Verification items for the finished model (mm, model axes). A direction names the side the tool comes from. Coordinates: 2 decimals unless noted, no trailing zeros. Order: outer loops, then holes, each group sorted by start corner. A loop starts at its lowest first (then second) coordinate and runs counter-clockwise, first axis right, second up. Notation, with made-up numbers: (54, -11) - (105, -11) arc R20 cw to (105, 2) - close; hole circle Ø9 at (41, 4.5). An arc over 180 degrees is marked (long way). One line per question, with ' | ' between items. Start each with the question number.
from build123d import *

# Parameters (mm, degrees)
SKETCH1_R           = 3
BOSS_EXTRUDE1_DEPTH = 29
CUT_EXTRUDE1_START  = -3
CUT_EXTRUDE1_DEPTH  = 3
FILLET1_R           = 1


with BuildPart() as part:
    # Sketch1 → Boss-Extrude1 (new body)
    with BuildSketch(Plane.XY):
        with Locations(Location((0, 0, 0), (0, 0, 180))):
            Circle(SKETCH1_R)
    extrude(amount=BOSS_EXTRUDE1_DEPTH)

    # Sketch3 → Cut-Extrude1 (cut)
    with BuildSketch(Plane.XY.offset(29).offset(CUT_EXTRUDE1_START)):
        with BuildLine():
            Line((-3, 0), (-1.5, 2.598076211))
            ThreePointArc((-1.5, 2.598076211), (-2.598076211, 1.5), (-3, 0))
        make_face()
        with BuildLine():
            Line((1.5, 2.598076211), (3, 0))
            ThreePointArc((3, 0), (2.598076211, 1.5), (1.5, 2.598076211))
        make_face()
        with BuildLine():
            Line((-1.5, 2.598076211), (1.5, 2.598076211))
            ThreePointArc((1.5, 2.598076211), (0, 3), (-1.5, 2.598076211))
        make_face()
        with BuildLine():
            ThreePointArc((-3, 0), (-2.598076211, -1.5), (-1.5, -2.598076211))
            Line((-1.5, -2.598076211), (-3, 0))
        make_face()
        with BuildLine():
            ThreePointArc((-1.5, -2.598076211), (0, -3), (1.5, -2.598076211))
            Line((1.5, -2.598076211), (-1.5, -2.598076211))
        make_face()
        with BuildLine():
            ThreePointArc((1.5, -2.598076211), (2.598076211, -1.5), (3, 0))
            Line((3, 0), (1.5, -2.598076211))
        make_face()
    cut_extrude1 = extrude(amount=CUT_EXTRUDE1_DEPTH, mode=Mode.SUBTRACT)

    # Mirror1: Cut-Extrude1 across plane
    add(cut_extrude1.mirror(Plane(origin=(0, 0, 14.5), x_dir=(1, 0, 0), z_dir=(0, 0, -1))), mode=Mode.SUBTRACT)

    # Sketch6 → Tap Drill for M3x0.5 Tap1 (revolve, cut)
    with BuildSketch(Plane(origin=(0, 0, 29), x_dir=(0, -1, 0), z_dir=(1, 0, 0))):
        Polygon((0, 0), (0, 5.751075774), (1.25, 5), (1.25, 0), align=None)
    tap_drill_for_m3x0_5_tap1 = revolve(axis=Axis((0, 0, 35.35), (0, 0, -1)), mode=Mode.SUBTRACT)

    # Mirror2: Tap Drill for M3x0.5 Tap1 across plane
    add(tap_drill_for_m3x0_5_tap1.mirror(Plane(origin=(0, 0, 14.5), x_dir=(1, 0, 0), z_dir=(0, 0, -1))), mode=Mode.SUBTRACT)

    # Fillet1
    # the kernel refuses this fillet: 1 mm, written as the material it takes off along each edge
    with BuildSketch(Plane(origin=(-1.5, 2.598076211, 26), x_dir=(-0.4999999999999951, -0.8660254037844416, 0), z_dir=(0, 0, 1)), Plane(origin=(3, 0, 26), x_dir=(-0.5000000000000018, 0.8660254037844377, 0), z_dir=(0, 0, 1)), Plane(origin=(1.5, 2.598076211, 26), x_dir=(-1, 0, 0), z_dir=(0, 0, 1)), Plane(origin=(1.5, -2.598076211, 26), x_dir=(0.4999999999999949, 0.8660254037844417, 0), z_dir=(0, 0, 1)), Plane(origin=(-1.5, -2.598076211, 26), x_dir=(1, 0, 0), z_dir=(0, 0, 1)), Plane(origin=(-3, 0, -1.443375673), x_dir=(0.500000000000007, -0.8660254037844346, 0), z_dir=(0, 0, 1)), Plane(origin=(3, 0, 3), x_dir=(-0.4999999999999955, -0.8660254037844413, 0), z_dir=(0, 0, -1)), Plane(origin=(1.5, -2.598076211, 3), x_dir=(-1, 0, 0), z_dir=(0, 0, -1)), Plane(origin=(-1.5, -2.598076211, 3), x_dir=(-0.5000000000000073, 0.8660254037844345, 0), z_dir=(0, 0, -1))) as fillet1_piece_1:
        with BuildLine():
            CenterArc((FILLET1_R * 0.57735026919, FILLET1_R), FILLET1_R, 210, 60)
            Line((-FILLET1_R * 0.288675134595, FILLET1_R * 0.5), (0, 0))
            Line((0, 0), (FILLET1_R * 0.57735026919, 0))
        make_face()
    extrude(amount=4.443375673, mode=Mode.SUBTRACT)
    with BuildSketch(Plane(origin=(-3, 0, 26), x_dir=(0.5000000000000109, 0.8660254037844323, 0), z_dir=(0, 0, 1)), Plane(origin=(-1.5, 2.598076211, 3), x_dir=(-0.4999999999999951, -0.8660254037844416, 0), z_dir=(0, 0, -1)), Plane(origin=(1.5, 2.598076211, 3), x_dir=(-1, 0, 0), z_dir=(0, 0, -1))) as fillet1_piece_2:
        with BuildLine():
            CenterArc((FILLET1_R * 0.57735026919, -FILLET1_R), FILLET1_R, 90, 60)
            Line((-FILLET1_R * 0.288675134595, -FILLET1_R * 0.5), (0, 0))
            Line((0, 0), (FILLET1_R * 0.57735026919, 0))
        make_face()
    extrude(amount=4.443375673, mode=Mode.SUBTRACT)


solid = part.part
Item 1: Section check B-B (y = 1.75). Record the cut outline in (x, z).
Item 2: Thickness scan on probe 1 along Y at (x, z) = (0, 1.2); probe 2 along Y at (x, z) = (0, 3.2); probe 3 along Z at (x, y) = (-2, -1.9). Record the ranges inside material, lowest first. Write a range as from..to.
Item 3: Section check A-A (z = 2). Record the cut outline in (x, y), then the cut area to 3 significant figures.
Item 4: Gauge pin test, flat ends, axial feed: pin 1 (2 mm diameter, centred on x = 0, y = 0, fed in from +Z); pin 2 (2 mm diameter, centred on x = 0, y = 0, fed in from -Z); pin 3 (0.9 mm diameter, centred on x = 0, z = 28, fed in from -Y). Record the tip position at first contact, or that the pin passes through.
Item 5: Set-up check for faces 1 (the flat face through (0, 2.598, 27)), 2 (the cylindrical face through (1.43, -2.46, 1.52)), 3 (the flat face through (0, -2.598, 27)): record each of +Z, -Z, +X, -X, +Y, -Y from which the full face is reachable in a straight line by a thin tool's end or side.
Completed:
1) outline: (-2.44, 3) - (-1.99, 3) - (-1.99, 0) - (1.99, 0) - (1.99, 3) - (2.44, 3) - (2.44, 26) - (1.99, 26) - (1.99, 29) - (-1.99, 29) - (-1.99, 26) - (-2.44, 26) - close
2) probe 1: y = -2.6..-1.25, 1.25..2.6 | probe 2: y = -3..-1.25, 1.25..3 | probe 3: z = 3..26
3) outline: (-2.71, -0.5) - (-1.79, -2.1) arc R1 ccw to (-0.92, -2.6) - (0.92, -2.6) arc R1 ccw to (1.79, -2.1) - (2.71, -0.5) arc R1 ccw to (2.71, 0.5) - (1.79, 2.1) arc R1 ccw to (0.92, 2.6) - (-0.92, 2.6) arc R1 ccw to (-1.79, 2.1) - (-2.71, 0.5) arc R1 ccw to start; hole circle Ø2.5 at (0, 0) | area: 18.2 mm^2
4) pin 1: stops at z = 23.85 | pin 2: stops at z = 5.15 | pin 3: stops at y = -2.6
5) face 1: +Z, +X, -X, +Y | face 2: -Z, +X, -Y | face 3: +Z, +X, -X, -Y
